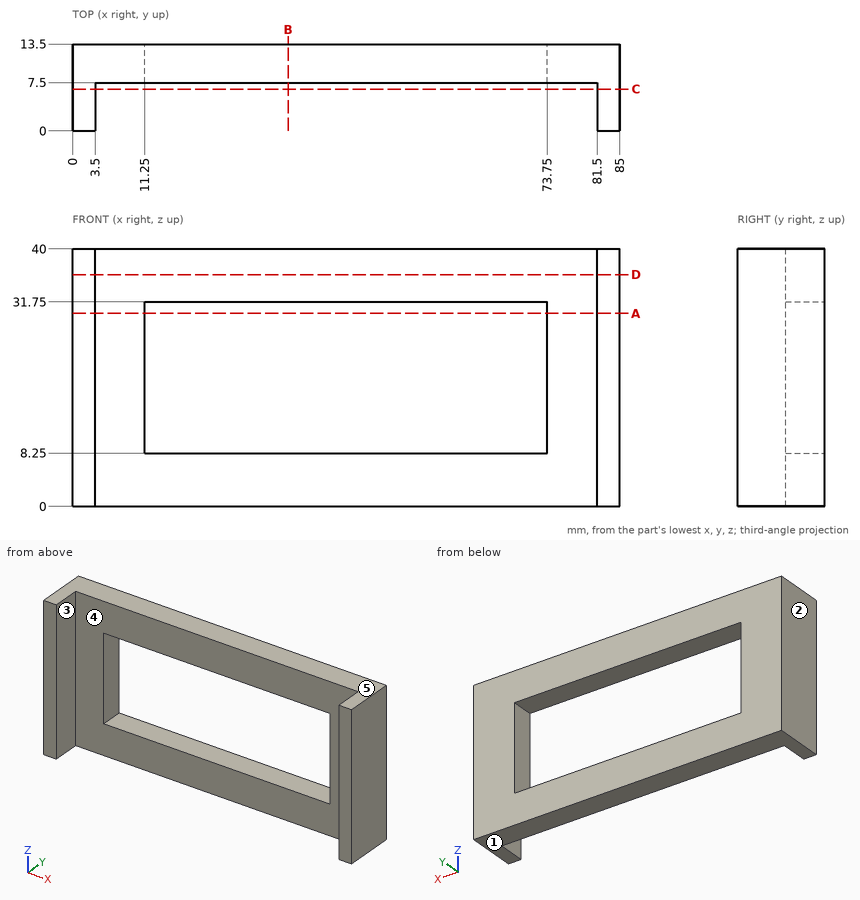
The figure shows three views and two pictorial views of one solid part (mm, origin at its lowest corner). Answer the questions. A direction names the side the tool comes from. Round coordinates to 2 decimals unless told otherwise and drop trailing zeros. Write each loop counter-clockwise with the first axis right and the second up, starting at its lowest first coordinate (ties: lowest second). Pieces come first, ordered by that corner, then holes. Notation, with made-up numbers: (-12, 66) -> (-8, 66) arc R22 ccw to (-8, 93) -> close; hole circle Ø5 at (48, 70.5). An arc over 180 degrees is marked (long way). Answer as a JSON object with one key per item and string values. Group by question number.
Q1. Which of the six approach directions +Z, -Z, +X, -X, +Y, -Y give full straight-line access (tool end or side, diameter ignored) to the marked faces 4 and 5?
Q2. Section B-B (x = 33.5) is taken. Write down the section's boundary in (y, z).
Q3. Section D-D (z = 36) is taken. Write down the section's boundary in (x, y).
Q4. This flat-tipped pin is pushed along its axis until it touches: pin 1 Ø8 at (x, z) = (75, 23) entering from -Y. Where does it stop, or does it pass through?
Q5. Determine the mould class of the marked faces 1, 2 and 3 for opening direction X: pulls with the +X half, pulls with the -X half, needs draft (parallel to the pull), parting line crosses it, or undercut.
Q6. Section C-C (y = 6.5) is taken. Write down the section's boundary in (x, z).
Q7. Straight lines are drawn through the part: line 1 along X through (y, z) = (10.5, 10); line 2 along Z through (x, y) = (45, 10); line 3 along X through (y, z) = (2.5, 28.5). For each, find the intervals that lie inside material, in ascending order.
Q8. Section A-A (z = 30) is taken. Write down the section's boundary in (x, y).
Check values:
{
 "1": {"face 4": "+Z, -Z, -Y", "face 5": "+Z, +X, -X, +Y, -Y"},
 "2": {"outline": "(7.5, 0) -> (13.5, 0) -> (13.5, 8.25) -> (7.5, 8.25) -> close; (7.5, 31.75) -> (13.5, 31.75) -> (13.5, 40) -> (7.5, 40) -> close"},
 "3": {"outline": "(0, 0) -> (3.5, 0) -> (3.5, 7.5) -> (81.5, 7.5) -> (81.5, 0) -> (85, 0) -> (85, 13.5) -> (0, 13.5) -> close"},
 "4": {"pin 1": "y = 7.5"},
 "5": {"face 1": "needs draft", "face 2": "pulls with the -X half", "face 3": "undercut"},
 "6": {"outline": "(0, 0) -> (3.5, 0) -> (3.5, 40) -> (0, 40) -> close; (81.5, 0) -> (85, 0) -> (85, 40) -> (81.5, 40) -> close"},
 "7": {"line 1": "0 to 11.25, 73.75 to 85", "line 2": "0 to 8.25, 31.75 to 40", "line 3": "0 to 3.5, 81.5 to 85"},
 "8": {"outline": "(0, 0) -> (3.5, 0) -> (3.5, 7.5) -> (11.25, 7.5) -> (11.25, 13.5) -> (0, 13.5) -> close; (73.75, 7.5) -> (81.5, 7.5) -> (81.5, 0) -> (85, 0) -> (85, 13.5) -> (73.75, 13.5) -> close"}
}
